Solid Edge part; units mm, degrees
sketch "Sketch1" plane through (0, 0, 0) normal (0, 0, 1) x (1, 0, 0)
  circle A0 centre (0, 0) radius 35
extrude "Protrusion1" add sketch "Sketch1" along normal blind 7
sketch "Sketch2" plane through (0, 0, 7) normal (0, 0, 1) x (1, 0, 0)
  line L0 (-17.5, -17.5) -> (17.5, -17.5)
  line L1 (17.5, -17.5) -> (17.5, 17.5)
  line L2 (17.5, 17.5) -> (-17.5, 17.5)
  line L3 (-17.5, 17.5) -> (-17.5, -17.5)
  dimension "D1" = 17.5
extrude "ExtrudedProtrusion_2" add sketch "Sketch2" along normal blind 63
sketch "Sketch3" plane through (0, 0, 70) normal (0, 0, 1) x (1, 0, 0)
  line L0 (-67.8, -24.7487) -> (24.7487, -24.7487)
  line L1 (24.7487, -24.7487) -> (24.7487, 24.7487)
  line L2 (24.7487, 24.7487) -> (-67.8, 24.7487)
  line L3 (-67.8, 24.7487) -> (-67.8, -24.7487)
  dimension "D1" = 24.7487
extrude "ExtrudedProtrusion_3" add sketch "Sketch3" along normal blind 7
sketch "Sketch4" plane through (-67.8, 0, 73.5) normal (-1, 0, 0) x (0, -1, 0)
  line L0 (-60, 3.5) -> (60, 3.5)
  line L1 (60, 3.5) -> (60, 100.35)
  line L2 (60, 100.35) -> (-60, 100.35)
  line L3 (-60, 100.35) -> (-60, 3.5)
  dimension "D1" = 60
extrude "ExtrudedProtrusion_4" add sketch "Sketch4" against normal blind 7
sketch "Sketch5" plane through (-60.8, 0, 125.425) normal (1, 0, 0) x (0, 1, 0)
  circle A0 centre (-50, 38.425) radius 1.35
  circle A1 centre (50, 38.425) radius 1.35
  dimension "D1" = 50
extrude "ExtrudedProtrusion_5" add sketch "Sketch5" along normal blind 111.6
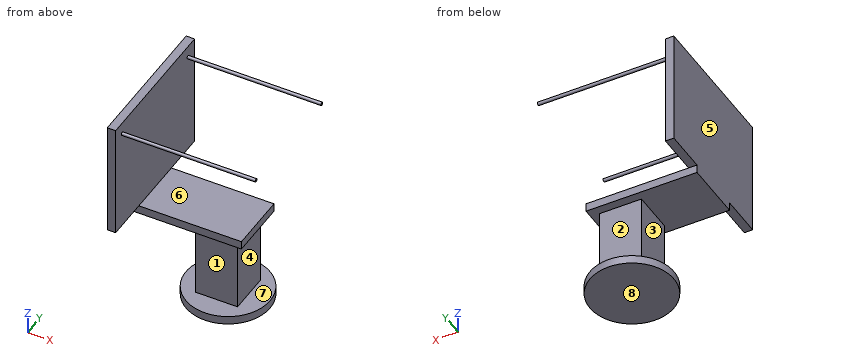
CAD build for the part. Positions are in the model's coordinates, mm. Face numbers are marked on the shaded views. A direction names the side the tool comes from. Coordinates: 2 decimals unless noted, no trailing zeros. Write each loop counter-clockwise with the first axis right and the second up, starting at its lowest first coordinate (ties: lowest second). Pieces come first, ordered by that corner, then holes. Notation, with made-up numbers: (73.25, -2.75) -> (126.25, -2.75) arc R10 ccw to (126.25, 13.25) -> close; hole circle Ø9 at (82, 22.5). An arc over 180 degrees is marked (long way). Use CSV: the item, a comma, the result in double quotes. Start each with the question number.
Item 1: Band-saw the part on C-C, the plane y = 0. Write the cut outline in (x, z), plus the area to 3 significant figures.
Item 2: Drop flat-ended pins along their axis: P1, Ø12, axis at x = -9, z = 62.5, coming from the +Y side; P2, Ø5.5, axis at x = -13.5, z = 75, coming from the -Y side; P3, Ø3.5, axis at x = -33.5, z = 75, coming from the +Y side. Give the stop position or say it passes through.
Item 3: Wall check: probe 1 along Z at (x, y) = (-5, -22); probe 2 along Z at (x, y) = (-54, -20.5); probe 3 along X at (y, z) = (14, 113). Give the ranges that are in metal, low to high.
Item 4: Band-saw the part on D-D, the plane z = 13.5. Write the cut outline in (x, y).
Item 5: Tool access for the marked faces 1, 2, 3, 4 and 5: list every direction of +Z, -Z, +X, -X, +Y, -Y with a clear straight run to the whole face (end or side of a thin tool).
Item 6: Two-plate mould, pull along Z, no slides. Class the marked faces 6, 7 and 8: +Z half, -Z half, draft (parallel to the pull), parting line (faces both ways), or undercut.
Item 7: Band-saw the part on A-A, the plane x = 0. Write the cut outline in (y, z).
Item 8: Band-saw the part on B-B, the plane y = -28. Write the cut outline in (x, z).
Response values:
1,outline,"(-67.8, 70) -> (-17.5, 70) -> (-17.5, 7) -> (-35, 7) -> (-35, 0) -> (35, 0) -> (35, 7) -> (17.5, 7) -> (17.5, 70) -> (24.75, 70) -> (24.75, 77) -> (-60.8, 77) -> (-60.8, 173.85) -> (-67.8, 173.85) -> close"
1,area,"4,020 mm2"
2,P1,"stops at y = 17.5"
2,P2,"stops at y = -24.75"
2,P3,"stops at y = 24.75"
3,probe 1,"z = 0 to 7, 70 to 77"
3,probe 2,"z = 70 to 77"
3,probe 3,"x = -67.8 to -60.8"
4,outline,"(-17.5, -17.5) -> (17.5, -17.5) -> (17.5, 17.5) -> (-17.5, 17.5) -> close"
5,face 1,"+X, -X, -Y"
5,face 2,"+X, -X, +Y"
5,face 3,"-X, +Y, -Y"
5,face 4,"+X, +Y, -Y"
5,face 5,"+Z, -Z, -X, +Y, -Y"
6,face 6,"+Z half"
6,face 7,"undercut"
6,face 8,"-Z half"
7,outline,"circle Ø2.7 at (-50, 163.85); (-35, 0) -> (35, 0) -> (35, 7) -> (17.5, 7) -> (17.5, 70) -> (24.75, 70) -> (24.75, 77) -> (-24.75, 77) -> (-24.75, 70) -> (-17.5, 70) -> (-17.5, 7) -> (-35, 7) -> close; circle Ø2.7 at (50, 163.85)"
8,outline,"(-67.8, 77) -> (-60.8, 77) -> (-60.8, 173.85) -> (-67.8, 173.85) -> close; (-21, 0) -> (21, 0) -> (21, 7) -> (-21, 7) -> close"
